Build history of the part. All positions in model axes, mm. A direction names the side the tool comes from. Round coordinates to 2 decimals unless told otherwise and drop trailing zeros. Loops run counter-clockwise (first coordinate to the right, second up) from the corner with the lowest first, then second, coordinate; pieces in that order, holes last. Notation, with made-up numbers: (-12, 41) - (40, 41) arc R22 cw to (40, 68) - close; hole circle Ø4 at (47, -26). An arc over 180 degrees is marked (long way). Answer as CSV lines item,"result". Start each with the question number.
```python
from build123d import *

# Parameters (mm, degrees)
SKETCH_R     = 3.95
SKETCH_R_2   = 1.6
PAD_DEPTH    = 11
CHAMFER_SIZE = 1
POCKET_DEPTH = 3


with BuildPart() as part:
    # Sketch → Pad (new body)
    with BuildSketch(Plane.XY):
        Circle(SKETCH_R)
        Circle(SKETCH_R_2, mode=Mode.SUBTRACT)
    extrude(amount=PAD_DEPTH)

    # Chamfer
    chamfer_edges = [part.edges().sort_by_distance(p)[0] for p in [
        (-3.95, 0, 0),
    ]]
    chamfer(chamfer_edges, length=CHAMFER_SIZE)

    # Sketch001 (on Face3 of Chamfer) → Pocket (cut)
    with BuildSketch(Plane.XY.offset(11)):
        Polygon((1.616581, 2.8), (-1.616581, 2.8), (-3.233162, 0), (-1.616581, -2.8), (1.616581, -2.8), (3.233162, 0), align=None)
    extrude(amount=-POCKET_DEPTH, mode=Mode.SUBTRACT)


solid = part.part
```
Q1. Two-plate mould, pull along Y, no slides. Class faces 1 (the flat face through (1.3, -1.3, 0)), 2 (the flat face through (-2.436, -1.38, 9.521)), 3 (the cylindrical face through (-3.135, -2.404, 5.93)): released by +Y, released by -Y, zero draft, split by the parting line, or undercut.
Q2. Pin check, flat tips, straight feed: pin 1 Ø1 at (x, y) = (2.5, -2.5) entering from -Z; pin 2 Ø1.5 at (y, z) = (-1, 10) entering from +X; pin 3 Ø1.9 at (x, y) = (0, 0) entering from -Z. Stop position of each tip, or through.
Q3. Band-saw the part on B-B, the plane z = 8.25. List the corners of the cut face in (x, y).
Q4. Wall check: probe 1 along Y at (x, z) = (0, 5.25); probe 2 along Z at (x, y) = (1, 2.25); probe 3 along X at (y, z) = (-0.5, 8.75). Give the ranges that are in metal, low to high. Write a range as [from, to].
Q5. Tool access for faces 4 (the flat face through (1.4, 1.3, 8)), 5 (the flat face through (-3, -1, 11)): list every direction of +Z, -Z, +X, -X, +Y, -Y with a clear straight run to the whole face (end or side of a thin tool).
Q6. Band-saw the part on C-C, the plane z = 4.25. List the corners of the cut face in (x, y).
Q7. Band-saw the part on A-A, the plane x = 0. List the corners of the cut face in (y, z).
Reported:
1,face 1,"zero draft"
1,face 2,"undercut"
1,face 3,"split by the parting line"
2,pin 1,"stops at z = 0.09"
2,pin 2,"stops at x = 3.94"
2,pin 3,"passes through"
3,outline,"circle Ø7.9 at (0, 0); hole (-3.23, 0) - (-1.62, -2.8) - (1.62, -2.8) - (3.23, 0) - (1.62, 2.8) - (-1.62, 2.8) - close"
4,probe 1,"y = [-3.95, -1.6], [1.6, 3.95]"
4,probe 2,"z = [0, 8]"
4,probe 3,"x = [-3.92, -2.94], [2.94, 3.92]"
5,face 4,"+Z"
5,face 5,"+Z, +X, -X, +Y, -Y"
6,outline,"circle Ø7.9 at (0, 0); hole circle Ø3.2 at (0, 0)"
7,outline,"(-3.95, 1) - (-2.95, 0) - (-1.6, 0) - (-1.6, 8) - (-2.8, 8) - (-2.8, 11) - (-3.95, 11) - close; (1.6, 0) - (2.95, 0) - (3.95, 1) - (3.95, 11) - (2.8, 11) - (2.8, 8) - (1.6, 8) - close"
